Autodesk Inventor part; units mm, degrees
ref_plane "YZ Plane" through (0, 0, 0) normal (1, 0, 0) x (0, 1, 0)
ref_plane "XZ Plane" through (0, 0, 0) normal (0, 1, 0) x (-1, 0, 0)
ref_plane "XY Plane" through (0, 0, 0) normal (0, 0, 1) x (1, 0, 0)
sketch "Эскиз1" plane through (0, 0, 0) normal (0, 0, 1) x (1, 0, 0)
  line L0 (-4.7, 2.25) -> (4.7, 2.25)
  line L1 (4.7, 2.25) -> (4.7, -2.25)
  line L2 (4.7, -2.25) -> (-4.7, -2.25)
  line L3 (-4.7, -2.25) -> (-4.7, 2.25)
  point P0 (0, 0)
  point P1 (-4.7, 0)
  point P2 (0, 2.25)
  dimension "d0" = 9.4
  dimension "d1" = 4.5
extrude "Выдавливание1" add sketch "Эскиз1" along normal mid plane 10.2
sketch "Эскиз3" plane through (0, 0, 5.1) normal (0, 0, 1) x (1, 0, 0)
  line L0 (-4.7, 2.25) -> (-4.7, -2.25)
  line L1 (-4.7, 0.75) -> (-2.9, 0.75)
  line L2 (-2.9, 0.75) -> (-2.9, 2.25)
  line L3 (4.7, 2.25) -> (-4.7, 2.25)
  line L4 (4.7, -2.25) -> (4.7, 2.25)
  line L5 (4.7, 0.75) -> (2.9, 0.75)
  line L6 (2.9, 0.75) -> (2.9, 2.25)
  point P0 (0, 0)
  dimension "d7" = 1.5
  dimension "d8" = 2.9
  dimension "d9" = 5.8
extrude "Выдавливание2" cut sketch "Эскиз3" against normal blind 10.2
sketch "Эскиз5" plane through (0, 0, 5.1) normal (0, 0, 1) x (1, 0, 0)
  line L0 (-4.7, -2.25) -> (4.7, -2.25)
  line L1 (-2.9, -2.25) -> (-4.7, -0.75)
  line L2 (-4.7, 0.75) -> (-4.7, -2.25)
  line L3 (4.7, -2.25) -> (4.7, 0.75)
  line L4 (4.7, -0.75) -> (2.9, -2.25)
  point P0 (0, 0)
  dimension "d15" = 1.5
  dimension "d16" = 2.9
  dimension "d17" = 5.8
extrude "Выдавливание3" cut sketch "Эскиз5" against normal blind 10.2
sketch "Эскиз6" plane through (-2.9, 2.25, -5.1) normal (0, 1, 0) x (1, 0, 0)
  point P0 (2.9, -5.1)
  point P1 (2.9, -5.1)
hole "Отверстие1" at (0, 2.25, 0) direction (0, -1, 0) diameter 5 end through all
thread "Резьба1"
chamfer "Фаска1" distance 0.2 angle 45 2 edges at (0, 2.25, -2.5) (0, -2.25, -2.5)
fillet "Сопряжение2" radius 0.1 2 edges at (2.9, 2.25, 0) (-2.9, 2.25, 0)
fillet "Сопряжение3" radius 0.3 2 edges at (-4.7, 0.75, 0) (4.7, 0.75, 0)
properties part number "COTS_GENERIC_20x20_M5_Nut" material "Сталь"
Design review of the part built by this model. Coordinates are the model's own, in mm. A direction names the side the tool comes from. Coordinates: 2 decimals unless noted, no trailing zeros. Loops run counter-clockwise (first coordinate to the right, second up) from the corner with the lowest first, then second, coordinate; pieces in that order, holes last.
Item 1: Add section C-C (y = 1.7). Write out the cut boundary in (x, z), and give its area (3 significant figures).
Completed:
outline: (-2.9, -5.1) - (2.9, -5.1) - (2.9, 5.1) - (-2.9, 5.1) - close; hole circle Ø5 at (0, 0)
area: 39.5 mm2
Item 2: Draft analysis for pull direction Z (two halves, no side actions). For faces 4 (the cylindrical face through (2.44, -0.03, -0.54)), 5 (the flat face through (2.6, -2.25, -1.2)), 6 (the flat face through (0, 0, -5.1)), state which applies: pulls with the +Z half, pulls with the -Z half, needs draft (parallel to the pull), parting line crosses it, or undercut.
Completed:
face 4: undercut
face 5: needs draft
face 6: pulls with the -Z half
Item 3: For faces 1 (the flat face through (4, 0.75, 0)), 2 (the flat face through (-4, 0.75, 0)), 3 (the flat face through (3.8, -1.5, 0.1)), list the 3-axis set-ups (+Z, -Z, +X, -X, +Y, -Y) from which the entire face can be reached by the end or side of a thin tool; tool diameter is ignored.
Completed:
face 1: +Z, -Z, +X, +Y
face 2: +Z, -Z, -X, +Y
face 3: +Z, -Z, +X, -Y
Item 4: Add section B-B (x = 0). Write out the cut boundary in (y, z), and give its area (3 significant figures).
Completed:
outline: (-2.25, -5.1) - (2.25, -5.1) - (2.25, -2.7) - (2.05, -2.5) - (-2.05, -2.5) - (-2.25, -2.7) - close; (-2.25, 2.7) - (-2.05, 2.5) - (2.05, 2.5) - (2.25, 2.7) - (2.25, 5.1) - (-2.25, 5.1) - close
area: 23.3 mm2
Item 5: Clearance check with flat-ended pins moving along their axes: pin 1 (1.1 mm diameter, centred on y = 1.5, z = -0.5, fed in from -X); pin 2 (1.7 mm diameter, centred on x = -4, z = -1, fed in from +Y); pin 3 (2 mm diameter, centred on x = -3, y = 1.5, fed in from -Z). State where each tip first meets the part, or that it passes through.
Completed:
pin 1: stops at x = -2.9
pin 2: stops at y = 0.75
pin 3: stops at z = -5.1
Item 6: Wall thickness on L1, parallel to Z at x = 0, y = 0.5; L2, parallel to X at y = 0.15, z = 0; L3, parallel to X at y = 1.1, z = 0: over which ranges is each line inside the solid? List them lowest first.
Completed:
L1: z = -5.1 to -2.5, 2.5 to 5.1
L2: x = -4.7 to -2.5, 2.5 to 4.7
L3: x = -2.9 to -2.5, 2.5 to 2.9
Item 7: Add section D-D (z = 3). Write out the cut boundary in (x, y), and give its area (3 significant figures).
Completed:
outline: (-4.7, -0.75) - (-2.9, -2.25) - (2.9, -2.25) - (4.7, -0.75) - (4.7, 0.45) arc R0.3 ccw to (4.4, 0.75) - (2.9, 0.75) - (2.9, 2.15) arc R0.1 ccw to (2.8, 2.25) - (-2.8, 2.25) arc R0.1 ccw to (-2.9, 2.15) - (-2.9, 0.75) - (-4.4, 0.75) arc R0.3 ccw to (-4.7, 0.45) - close
area: 34.2 mm2
Item 8: Add section A-A (z = 0). Write out the cut boundary in (x, y).
Completed:
outline: (-4.7, -0.75) - (-2.9, -2.25) - (-2.7, -2.25) - (-2.5, -2.05) - (-2.5, 2.05) - (-2.7, 2.25) - (-2.8, 2.25) arc R0.1 ccw to (-2.9, 2.15) - (-2.9, 0.75) - (-4.4, 0.75) arc R0.3 ccw to (-4.7, 0.45) - close; (2.5, -2.05) - (2.7, -2.25) - (2.9, -2.25) - (4.7, -0.75) - (4.7, 0.45) arc R0.3 ccw to (4.4, 0.75) - (2.9, 0.75) - (2.9, 2.15) arc R0.1 ccw to (2.8, 2.25) - (2.7, 2.25) - (2.5, 2.05) - close
